For this review, take the finished solid that the model builds, in its own axes (mm). A direction names the side the tool comes from. Coordinates: 2 decimals unless noted, no trailing zeros. Write each loop counter-clockwise with the first axis right and the second up, starting at its lowest first coordinate (ties: lowest second). Pieces come first, ordered by that corner, then holes. Notation, with made-up numbers: (17.25, 4) - (27.25, 4) arc R17 cw to (27.25, 9) - close; hole circle Ø8 at (50.5, -1). An arc over 180 degrees is marked (long way). Write each question's results on one line, items separated by ' | '.
Autodesk Inventor part; units mm, degrees
ref_plane "YZ Plane" through (0, 0, 0) normal (1, 0, 0) x (0, 1, 0)
ref_plane "XZ Plane" through (0, 0, 0) normal (0, 1, 0) x (-1, 0, 0)
ref_plane "XY Plane" through (0, 0, 0) normal (0, 0, 1) x (1, 0, 0)
sketch "草圖1" plane through (0, 0, 0) normal (0, 0, 1) x (1, 0, 0)
  line L0 (0, 0) -> (150, 4)
  line L1 (150, 4) -> (150, -6)
  line L2 (150, -6) -> (0, -6)
  line L3 (0, -6) -> (0, 0)
  dimension "d0" = 10
  dimension "d1" = 6
  dimension "d2" = 150
extrude "擠出1" add sketch "草圖1" along normal blind 25
sketch "草圖2" plane through (0, -6, 0) normal (0, -1, 0) x (1, 0, 0)
  circle A0 centre (50, 12.5) radius 5
  circle A1 centre (130, 12.5) radius 5
  line L0 (0, 25) -> (150, 25)
  line L1 (150, 0) -> (150, 25)
  point P0 (0, 0)
  dimension "d5" = 12.5
  dimension "d6" = 10
  dimension "d7" = 10
  dimension "d8" = 80
  dimension "d9" = 20
extrude "擠出2" add sketch "草圖2" along normal blind 21
sketch "草圖3" plane through (0, -6, 0) normal (-1, 0, 0) x (0, 0, 1)
  line L0 (0, 0) -> (0, 6) construction
  line L1 (0, 0) -> (25, 0) construction
  line L2 (25, 6) -> (25, 0) construction
  line L3 (0, 6) -> (25, 6) construction
  line L4 (21, 6) -> (4, 6)
  line L5 (0, 6) -> (25, 6)
  arc A0 (4.2386, 6) -> (20.7614, 6) centre (12.5, 8) ccw
  dimension "d23" = 17
  dimension "d25" = 2
sketch "草圖4" plane through (150, -6, 0) normal (1, 0, 0) x (0, 0, -1)
  line L0 (-21.5, 11) -> (-3.5, 11)
  arc A0 (-21.275, 11) -> (-3.725, 11) centre (-12.5, 13) ccw
  line L1 (0, 10) -> (0, 0)
  dimension "d19" = 18
  dimension "d21" = 2
  dimension "d22" = 12.5
sketch "草圖5" plane through (0, 0, 25) normal (-0.0267, 0.9996, 0) x (0.9996, 0.0267, 0)
  line L0 (150.0533, 25) -> (150.0533, 0)
  line L1 (150.0533, 12.5) -> (0, 12.5)
  line L2 (0, 25) -> (0, 0)
loft "斷面混成2" cut profiles "草圖4", "草圖3"
properties part number "滑軌3"
Q1. For faces 5 (the face through (130, -27, 13)), 6 (the face through (46.315, -16.353, 9.121)), list the 3-axis set-ups (+Z, -Z, +X, -X, +Y, -Y) from which the entire face can be reached by the end or side of a thin tool; tool diameter is ignored.
Results found:
face 5: +Z, -Z, +X, -X, -Y | face 6: -Y
Q2. Mouldability with a two-part tool opening along X and no side actions: class faces 1 (the face through (0, -4, 3)), 2 (the face through (150, -3, 12)), 3 (the face through (134.77, -16.35, 11)), 4 (the face through (76, -6, 12)) as pulls with the +X half, pulls with the -X half, needs draft (parallel to the pull), parting line crosses it, or undercut.
Results found:
face 1: pulls with the -X half | face 2: pulls with the +X half | face 3: undercut | face 4: undercut
Q3. For pin 1 (1 mm diameter, centred on x = 131.5, y = -7.5, fed in from +Z); pin 2 (2 mm diameter, centred on x = 131.5, z = 20, fed in from -Y); pin 3 (1 mm diameter, centred on y = -18.5, z = 5.5, fed in from -X); pin 4 (10 mm diameter, centred on x = 101.5, z = 9, fed in from +Y), all flat-tipped, find the tip position at first contact; note any pin that passes through.
Results found:
pin 1: z = 17.4 | pin 2: y = -6 | pin 3: through | pin 4: y = 2.73
Q4. Wall thickness on line 1 along Z through (x, y) = (71, 1.5); line 2 along X through (y, z) = (-22, 11); line 3 along Z through (x, y) = (29.5, 0): over which ranges is each line inside the solid? List them lowest first. Write a range as from..to.
Results found:
line 1: 0..4.25, 20.75..25 | line 2: 45.23..54.77, 125.23..134.77 | line 3: 0..4.44, 20.56..25
Q5. Take a section at A-A on y = -22. State the section outline as (x, z) points, plus the area to 3 significant figures.
Results found:
outline: circle Ø10 at (50, 12.5); circle Ø10 at (130, 12.5) | area: 157 mm2
